For this review, take the finished solid that the model builds, in its own axes (mm). A direction names the side the tool comes from. Round coordinates to 2 decimals unless told otherwise and drop trailing zeros. Write each loop counter-clockwise with the first axis right and the second up, starting at its lowest first coordinate (ties: lowest second). Pieces come first, ordered by that corner, then holes. Notation, with made-up numbers: M -3.75,59.25 L 40.25,59.25 A29 ccw 40.25,93.25 Z; hole C 36,-38.75 d10. An arc over 180 degrees is marked long. One line per question, with ' | ' between items.
```python
from build123d import *

# Parameters (mm, degrees)
BOSS_EXTRUDE1_DEPTH = 15
BOSS_EXTRUDE2_DEPTH = 3
SKETCH3_W           = 8
SKETCH3_H           = 12
CUT_EXTRUDE1_DEPTH  = 10
CUT_EXTRUDE3_DEPTH  = 10


with BuildPart() as part:
    # Sketch1 → Boss-Extrude1 (new body)
    with BuildSketch(Plane(origin=(0, 0, 0), x_dir=(1, 0, 0), z_dir=(0, 1, 0))):
        with BuildLine():
            Line((1.5, 0), (30.5, 0))
            ThreePointArc((30.5, 0), (31.560660172, 0.439339828), (32, 1.5))
            Line((32, 1.5), (32, 10.5))
            ThreePointArc((32, 10.5), (31.560660172, 11.560660172), (30.5, 12))
            Line((30.5, 12), (1.5, 12))
            ThreePointArc((1.5, 12), (0.439339828, 11.560660172), (0, 10.5))
            Line((0, 10.5), (0, 1.5))
            ThreePointArc((0, 1.5), (0.439339828, 0.439339828), (1.5, 0))
        make_face()
    extrude(amount=BOSS_EXTRUDE1_DEPTH)

    # Sketch2 → Boss-Extrude2 (add)
    with BuildSketch(Plane(origin=(0, 15, 0), x_dir=(1, 0, 0), z_dir=(0, 1, 0))):
        with BuildLine():
            Line((1.5, -2), (30.5, -2))
            ThreePointArc((30.5, -2), (32.974873734, -0.974873734), (34, 1.5))
            Line((34, 1.5), (34, 10.5))
            ThreePointArc((34, 10.5), (32.974873734, 12.974873734), (30.5, 14))
            Line((30.5, 14), (1.5, 14))
            ThreePointArc((1.5, 14), (-0.974873734, 12.974873734), (-2, 10.5))
            Line((-2, 10.5), (-2, 1.5))
            ThreePointArc((-2, 1.5), (-0.974873734, -0.974873734), (1.5, -2))
        make_face()
        with BuildLine():
            ThreePointArc((32, 10.5), (31.560660172, 11.560660172), (30.5, 12))
            Line((30.5, 12), (1.5, 12))
            ThreePointArc((1.5, 12), (0.439339828, 11.560660172), (0, 10.5))
            Line((0, 10.5), (0, 1.5))
            ThreePointArc((0, 1.5), (0.439339828, 0.439339828), (1.5, 0))
            Line((1.5, 0), (30.5, 0))
            ThreePointArc((30.5, 0), (31.560660172, 0.439339828), (32, 1.5))
            Line((32, 1.5), (32, 10.5))
        make_face(mode=Mode.SUBTRACT)
        with BuildLine():
            Line((32, 1.5), (32, 10.5))
            ThreePointArc((32, 10.5), (31.560660172, 11.560660172), (30.5, 12))
            Line((30.5, 12), (1.5, 12))
            ThreePointArc((1.5, 12), (0.439339828, 11.560660172), (0, 10.5))
            Line((0, 10.5), (0, 1.5))
            ThreePointArc((0, 1.5), (0.439339828, 0.439339828), (1.5, 0))
            Line((1.5, 0), (30.5, 0))
            ThreePointArc((30.5, 0), (31.560660172, 0.439339828), (32, 1.5))
        make_face()
    extrude(amount=BOSS_EXTRUDE2_DEPTH)

    # Sketch3 → Cut-Extrude1 (cut)
    with BuildSketch(Plane.XZ):
        with Locations((16, -6)):
            Rectangle(SKETCH3_W, SKETCH3_H)
    extrude(amount=-CUT_EXTRUDE1_DEPTH, mode=Mode.SUBTRACT)

    # Sketch4 → Cut-Extrude3 (cut)
    with BuildSketch(Plane.XZ):
        with BuildLine():
            Line((8.5, 0), (1.5, 0))
            ThreePointArc((1.5, 0), (0.439339828, -0.439339828), (0, -1.5))
            Line((0, -1.5), (0, -10.5))
            ThreePointArc((0, -10.5), (0.439339828, -11.560660172), (1.5, -12))
            Line((1.5, -12), (8.5, -12))
            Line((8.5, -12), (8.5, 0))
        make_face()
        with BuildLine():
            Line((23.5, -12), (30.5, -12))
            ThreePointArc((30.5, -12), (31.560660172, -11.560660172), (32, -10.5))
            Line((32, -10.5), (32, -1.5))
            ThreePointArc((32, -1.5), (31.560660172, -0.439339828), (30.5, 0))
            Line((30.5, 0), (23.5, 0))
            Line((23.5, 0), (23.5, -12))
        make_face()
    extrude(amount=-CUT_EXTRUDE3_DEPTH, mode=Mode.SUBTRACT)


solid = part.part
```
Item 1: Take a section at B-B (x = 7.5). Write out the cut boundary in (y, z), then the cut area to 3 significant figures.
Results:
outline: M 10,-12 L 15,-12 L 15,-14 L 18,-14 L 18,2 L 15,2 L 15,0 L 10,0 Z | area: 108 mm2
Item 2: Take a section at A-A (y = 9). Write out the cut boundary in (x, z), then the cut area to 3 significant figures.
Results:
outline: M 8.5,-12 L 12,-12 L 12,0 L 8.5,0 Z; M 20,-12 L 23.5,-12 L 23.5,0 L 20,0 Z | area: 84.0 mm2
Item 3: To check wall thickness, follow line 1 along X through (y, z) = (4, -1.5); line 2 along Y through (x, z) = (29.5, -11.75); line 3 along Y through (x, z) = (5, 0.5). State the ranges of each line that lie inside material, in increasing order. Write a range as from..to.
Results:
line 1: 8.5..12, 20..23.5 | line 2: 10..18 | line 3: 15..18
Item 4: Machinability: for faces 1 (the face through (23.5, 5, -6)), 2 (the face through (4, 10, -6)), 3 (the face through (12, 5, -6)), which of the approach directions +Z, -Z, +X, -X, +Y, -Y give a long, thin tool a straight path to every point of the face, cutting with its end or side? Answer none if there is none.
Results:
face 1: +Z, -Z, +X, -Y | face 2: +Z, -Z, -X, -Y | face 3: +Z, -Z, -Y
Item 5: Mouldability with a two-part tool opening along X and no side actions: class faces 4 (the face through (16, 11, 0)), 5 (the face through (20, 5, -6)), 6 (the face through (31.57, 12.46, -11.55)), 7 (the face through (-2, 16, -6)) as +X half, -X half, draft (parallel to the pull), parting line (faces both ways), or undercut.
Results:
face 4: draft | face 5: undercut | face 6: +X half | face 7: -X half
Item 6: Take a section at C-C (z = -9). Write out the cut boundary in (x, y), then the cut area to 3 significant figures.
Results:
outline: M -2,15 L 0,15 L 0,10 L 8.5,10 L 8.5,0 L 12,0 L 12,10 L 20,10 L 20,0 L 23.5,0 L 23.5,10 L 32,10 L 32,15 L 34,15 L 34,18 L -2,18 Z | area: 338 mm2
Item 7: Insertion check: pin 1 Ø8 at (y, z) = (3.5, -5) entering from +X; pin 2 Ø2 at (x, y) = (12, 12) entering from -Z; pin 3 Ø2 at (y, z) = (12.5, -8.5) entering from -X. Each pin has a flat end and moves straight along its axis. Give the tip position at first contact, or say it passes through.
Results:
pin 1: x = 23.5 | pin 2: z = -12 | pin 3: x = 0
Item 8: Take a section at D-D (y = 13.25). Write out the cut boundary in (x, z), then the cut area to 3 significant figures.
Results:
outline: M 0,-10.5 A1.5 ccw 1.5,-12 L 30.5,-12 A1.5 ccw 32,-10.5 L 32,-1.5 A1.5 ccw 30.5,0 L 1.5,0 A1.5 ccw 0,-1.5 Z | area: 382 mm2
